Answer from the drawing. Dimensions are ordinates in mm from the lowest x, y and z of the part. Give positions to 0.01 mm unless a question says otherwise; leave off trailing zeros. Write each loop counter-clockwise with the first axis right and the second up, starting at its lowest first coordinate (ties: lowest second). Pieces come first, ordered by that corner, then holes. Notation, with made-up numbers: (-16, 6.25) -> (2, 6.25) arc R20 ccw to (2, 28.25) -> close; hole circle Ø10 at (-19, 3.25). An arc over 180 degrees is marked (long way). Use a Markdown table: item, result. Add a question column.
Q1. Each of these flat-tipped pins is pushed along its axis until it touches: pin 1 Ø1.5 at (x, y) = (110.5, 1.5) entering from -Z; pin 2 Ø1.5 at (x, y) = (120.5, 1) entering from -Z; pin 3 Ø1 at (x, y) = (136.5, 1) entering from -Z. Where does it stop, or does it pass through?
Q2. Section C-C, the plane x = 17.5 is taken. Give the vertices of the cut face in (y, z).
Q3. Section D-D, the plane z = 183 is taken. Give the vertices of the cut face in (x, y) (1 decimal).
Q4. Section B-B, the plane z = 93.5 is taken. Give the vertices of the cut face in (x, y).
Q5. Consider line 1 (Z direction, x = 170.5, y = 1.75) (1 decimal); line 2 (Z direction, x = 123, y = 2.15) (1 decimal); line 3 (Z direction, x = 12.5, y = 0.65) (1 decimal). Determine where each line is inside the solid, lowest interval first.
Q6. Section A-A, the plane x = 56.5 is taken. Give the vertices of the cut face in (y, z).
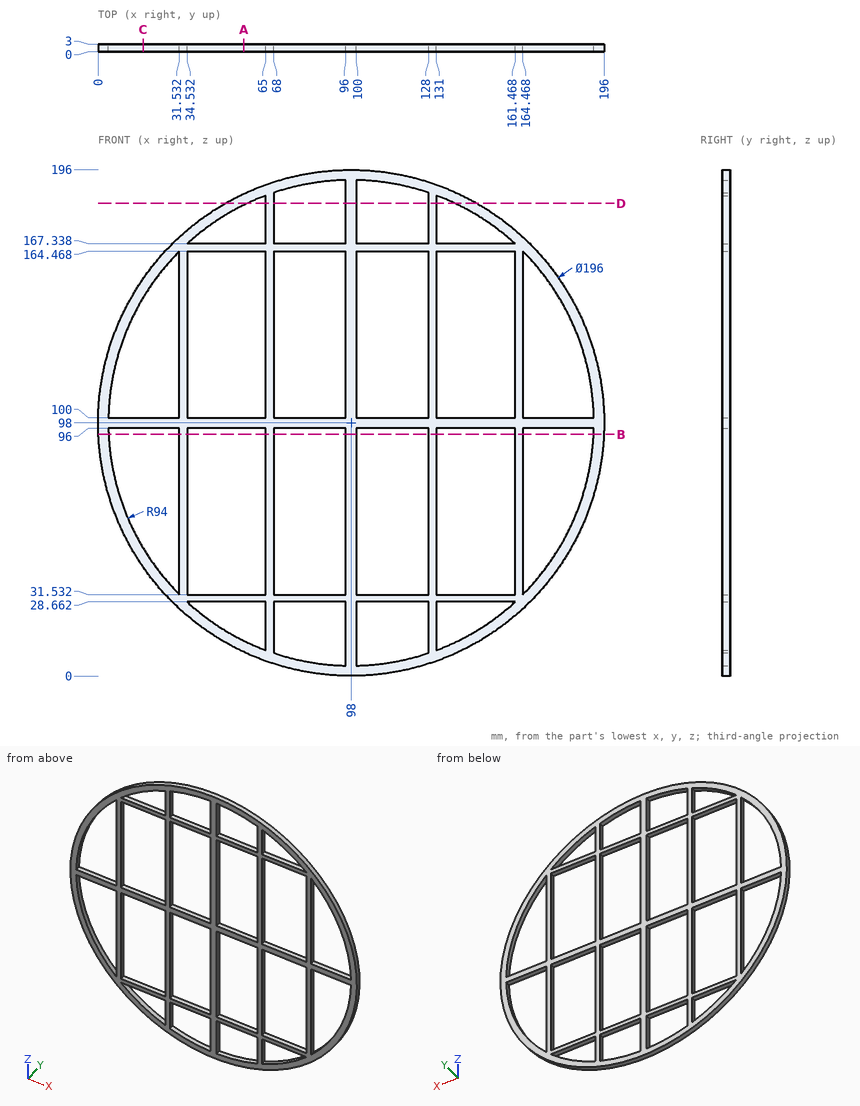
Result set:
| question | item | result |
|---|---|---|
| 1 | pin 1 | stops at z = 0.71 |
| 1 | pin 2 | stops at z = 2.44 |
| 1 | pin 3 | stops at z = 7.67 |
| 2 | outline | (0, 42.11) -> (3, 42.11) -> (3, 49.46) -> (0, 49.46) -> close; (0, 96) -> (3, 96) -> (3, 100) -> (0, 100) -> close; (0, 146.54) -> (3, 146.54) -> (3, 153.89) -> (0, 153.89) -> close |
| 3 | outline | (49.2, 0) -> (57.9, 0) -> (57.9, 3) -> (49.2, 3) -> close; (65, 0) -> (68, 0) -> (68, 3) -> (65, 3) -> close; (96, 0) -> (100, 0) -> (100, 3) -> (96, 3) -> close; (128, 0) -> (131, 0) -> (131, 3) -> (128, 3) -> close; (138.1, 0) -> (146.8, 0) -> (146.8, 3) -> (138.1, 3) -> close |
| 4 | outline | (0.1, 0) -> (4.11, 0) -> (4.11, 3) -> (0.1, 3) -> close; (31.53, 0) -> (34.53, 0) -> (34.53, 3) -> (31.53, 3) -> close; (65, 0) -> (68, 0) -> (68, 3) -> (65, 3) -> close; (96, 0) -> (100, 0) -> (100, 3) -> (96, 3) -> close; (128, 0) -> (131, 0) -> (131, 3) -> (128, 3) -> close; (161.47, 0) -> (164.47, 0) -> (164.47, 3) -> (161.47, 3) -> close; (191.89, 0) -> (195.9, 0) -> (195.9, 3) -> (191.89, 3) -> close |
| 5 | line 1 | z = 32.1 to 38.2, 96 to 100, 157.8 to 163.9 |
| 5 | line 2 | z = 3.2 to 7.4, 28.7 to 31.5, 96 to 100, 164.5 to 167.3, 188.6 to 192.8 |
| 5 | line 3 | z = 50.1 to 58.9, 96 to 100, 137.1 to 145.9 |
| 6 | outline | (0, 9.22) -> (3, 9.22) -> (3, 13.66) -> (0, 13.66) -> close; (0, 28.66) -> (3, 28.66) -> (3, 31.53) -> (0, 31.53) -> close; (0, 96) -> (3, 96) -> (3, 100) -> (0, 100) -> close; (0, 164.47) -> (3, 164.47) -> (3, 167.34) -> (0, 167.34) -> close; (0, 182.34) -> (3, 182.34) -> (3, 186.78) -> (0, 186.78) -> close |
